from build123d import *

# Parameters (mm, degrees)
SKETCH2_W                  = 23.9522
SKETCH2_H                  = 45.7962
SKETCH2_R                  = 2.2606
SKETCH2_R_2                = 1.016
BOSS_EXTRUDE1_DEPTH        = 6.35
SKETCH4_W                  = 21.4122
SKETCH4_H                  = 43.2562
CUT_EXTRUDE1_DEPTH         = 6.223
CUT_EXTRUDE3_DEPTH         = 2.54
CUT_EXTRUDE5_DEPTH         = 1.27
BOSS_EXTRUDE3_DEPTH        = 6.223
BOSS_EXTRUDE15_OUTLINE_W   = 23.9522
BOSS_EXTRUDE15_OUTLINE_H   = 30.5562
BOSS_EXTRUDE15_OUTLINE_R   = 2.2606
BOSS_EXTRUDE15_OUTLINE_R_2 = 1.016
BOSS_EXTRUDE15_DEPTH       = 1.27
SKETCH14_R                 = 1.190625
CUT_EXTRUDE6_DEPTH         = 1.27


# Read off the part's stored shape, not the designer's step: Boss-Extrude15
with BuildPart() as part:
    # Sketch2 → Boss-Extrude1 (new body)
    with BuildSketch(Plane.XY):
        Rectangle(SKETCH2_W, SKETCH2_H)
        with Locations((0, -8.7249)):
            Circle(SKETCH2_R, mode=Mode.SUBTRACT)
        with Locations((0, 13.4747)):
            Circle(SKETCH2_R_2, mode=Mode.SUBTRACT)
        with BuildLine():
            Line((8.361518313, 5.139100055), (5.725634689, 6.065681687))
            ThreePointArc((5.725634689, 6.065681687), (4.333034634, 5.3975), (5.001216321, 4.004899945))
            Line((5.001216321, 4.004899945), (7.637099945, 3.078318313))
            ThreePointArc((7.637099945, 3.078318313), (9.0297, 3.7465), (8.361518313, 5.139100055))
        make_face(mode=Mode.SUBTRACT)
    extrude(amount=BOSS_EXTRUDE1_DEPTH)

    # Sketch4 → Cut-Extrude1 (cut)
    with BuildSketch(Plane.XY.offset(6.35)):
        Rectangle(SKETCH4_W, SKETCH4_H)
    extrude(amount=-CUT_EXTRUDE1_DEPTH, mode=Mode.SUBTRACT)

    # Sketch6 → Cut-Extrude3 (cut)
    with BuildSketch(Plane.ZY.offset(11.9761)):
        Polygon((4.826, -14.5669), (2.6162, -14.5669), (2.6162, 4.9911), (6.35, 4.9911), (6.35, -18.7833), (4.826, -18.7833), align=None)
    extrude(amount=-CUT_EXTRUDE3_DEPTH, mode=Mode.SUBTRACT)

    # Sketch8 → Cut-Extrude5 (cut)
    with BuildSketch(Plane(origin=(11.9761, 0, 0), x_dir=(0, 0, -1), z_dir=(1, 0, 0))):
        Polygon((-6.35, -18.7833), (-4.826, -18.7833), (-4.826, -14.5669), (-2.8956, -14.5669), (-2.8956, -6.0325), (0, -5.1181), (0, 13.4239), (-6.35, 13.3731), align=None)
    extrude(amount=-CUT_EXTRUDE5_DEPTH, mode=Mode.SUBTRACT)

    # Sketch10 → Boss-Extrude3 (add)
    with BuildSketch(Plane.XY.offset(0.127)):
        with BuildLine():
            ThreePointArc((-10.7061, 20.3581), (-9.808074388, 20.730074388), (-9.4361, 21.6281))
            Line((-9.4361, 21.6281), (-10.7061, 21.6281))
            Line((-10.7061, 21.6281), (-10.7061, 20.3581))
        make_face()
        with BuildLine():
            ThreePointArc((9.4361, 21.6281), (9.808074388, 20.730074388), (10.7061, 20.3581))
            Line((10.7061, 20.3581), (10.7061, 21.6281))
            Line((10.7061, 21.6281), (9.4361, 21.6281))
        make_face()
        with BuildLine():
            ThreePointArc((-9.4361, -21.6281), (-9.808074388, -20.730074388), (-10.7061, -20.3581))
            Line((-10.7061, -20.3581), (-10.7061, -21.6281))
            Line((-10.7061, -21.6281), (-9.4361, -21.6281))
        make_face()
        with BuildLine():
            Line((10.7061, -21.6281), (10.7061, -20.3581))
            ThreePointArc((10.7061, -20.3581), (9.808074388, -20.730074388), (9.4361, -21.6281))
            Line((9.4361, -21.6281), (10.7061, -21.6281))
        make_face()
    extrude(amount=BOSS_EXTRUDE3_DEPTH)

    # Boss-Extrude15 outline → Boss-Extrude15 (add)
    with BuildSketch(Plane(origin=(0, 0, 0), x_dir=(-1, 0, 0), z_dir=(0, 0, -1))):
        with Locations((0, 2.54)):
            Rectangle(BOSS_EXTRUDE15_OUTLINE_W, BOSS_EXTRUDE15_OUTLINE_H)
        with Locations((0, -8.7249)):
            Circle(BOSS_EXTRUDE15_OUTLINE_R, mode=Mode.SUBTRACT)
        with BuildLine():
            ThreePointArc((-7.637099945, 3.078318313), (-9.0297, 3.7465), (-8.361518313, 5.139100055))
            Line((-8.361518313, 5.139100055), (-5.725634689, 6.065681687))
            ThreePointArc((-5.725634689, 6.065681687), (-4.333034634, 5.3975), (-5.001216321, 4.004899945))
            Line((-5.001216321, 4.004899945), (-7.637099945, 3.078318313))
        make_face(mode=Mode.SUBTRACT)
        with Locations((0, 13.4747)):
            Circle(BOSS_EXTRUDE15_OUTLINE_R_2, mode=Mode.SUBTRACT)
    extrude(amount=BOSS_EXTRUDE15_DEPTH)

    # Sketch14 → Cut-Extrude6 (cut)
    with BuildSketch(Plane.ZY.offset(11.9761)):
        with Locations((6.35, 11.528736377)):
            Circle(SKETCH14_R)
    extrude(amount=-CUT_EXTRUDE6_DEPTH, mode=Mode.SUBTRACT)


solid = part.part
CAD build for the part. Positions are in the model's coordinates, mm. A direction names the side the tool comes from. Give positions to 0.01 mm unless a question says otherwise; leave off trailing zeros. Loops run counter-clockwise (first coordinate to the right, second up) from the corner with the lowest first, then second, coordinate; pieces in that order, holes last. Notation, with made-up numbers: M -36.5,63 L 8.5,63 A24 ccw 8.5,85 Z; hole C 39,-13 d4. An arc over 180 degrees is marked long. One line per question, with ' | ' between items. Start each with the question number.
1. Saw through at B-B on y = 15.5. Give the cut face in (x, z), plus the area to 3 significant figures.
2. Two-plate mould, pull along Y, no slides. Class faces 1 (the face through (11, -14.567, 4)), 2 (the face through (0, 17.818, -1)), 3 (the face through (0, -22, 6.35)): pulls with the +Y half, pulls with the -Y half, needs draft (parallel to the pull), parting line crosses it, or undercut.
3. 3-axis set-ups, long thin cutter, end or side, ignore diameter. For faces 4 (the face through (11.976, 0, -1)), 5 (the face through (11.35, -5.582, 1.468)), 6 (the face through (-11, -5, 2.616)), 7 (the face through (-11, -17, 4.826)), 8 (the face through (10.706, 17, 3)): which of +Z, -Z, +X, -X, +Y, -Y reach the whole face in a straight line?
4. Saw through at A-A on x = 0. Give the cut face in (y, z), plus the area to 3 significant figures.
5. Probe L1, parallel to Y at x = 0, z = -0.7; L2, parallel to Y at x = -3.5, z = 0.5; L3, parallel to Y at x = -10.75, z = 5.5. List the from-to ranges inside material, lowest first. Write a range as from..to.
6. Saw through at C-C on z = 3.5. Give the cut face in (x, y), plus the area to 3 significant figures.
7. Flat gauge pins, fed straight in: pin 1 (1.9 mm diameter, centred on y = 3, z = 3.5, fed in from +X); pin 2 (3.5 mm diameter, centred on x = 0, y = 13.47, fed in from +Z); pin 3 (0.6 mm diameter, centred on x = -11, y = -5.5, fed in from +Z). Where does each tip first touch, or does it go through?
8. Saw through at D-D on x = -6. Give the cut face in (y, z), plus the area to 3 significant figures.
Result sheet:
1) outline: M -11.98,-1.27 L 11.98,-1.27 L 11.98,6.35 L 10.71,6.35 L 10.71,0.13 L -10.71,0.13 L -10.71,6.35 L -11.98,6.35 Z | area: 49.3 mm^2
2) face 1: undercut | face 2: pulls with the +Y half | face 3: needs draft
3) face 4: +Z, -Z, +X, +Y, -Y | face 5: +Z, +X | face 6: +Z, -X | face 7: +Z, +X, -X | face 8: +Z
4) outline: M -22.9,0 L -12.74,0 L -12.74,-1.27 L -10.99,-1.27 L -10.99,0.13 L -21.63,0.13 L -21.63,6.35 L -22.9,6.35 Z; M -6.46,-1.27 L 12.46,-1.27 L 12.46,0.13 L -6.46,0.13 Z; M 14.49,-1.27 L 17.82,-1.27 L 17.82,0 L 22.9,0 L 22.9,6.35 L 21.63,6.35 L 21.63,0.13 L 14.49,0.13 Z | area: 51.3 mm^2
5) L1: y = -12.74..-10.99, -6.46..12.46, 14.49..17.82 | L2: y = -22.9..-21.63, 21.63..22.9 | L3: y = -22.9..-18.78, 4.99..10.7, 12.36..22.9
6) outline: M -11.98,-22.9 L 11.98,-22.9 L 11.98,-14.57 L 10.71,-14.57 L 10.71,-20.36 A1.27 ccw 9.44,-21.63 L -9.44,-21.63 A1.27 ccw -10.71,-20.36 L -10.71,-14.57 L -11.98,-14.57 Z; M -11.98,4.99 L -10.71,4.99 L -10.71,20.36 A1.27 ccw -9.44,21.63 L 9.44,21.63 A1.27 ccw 10.71,20.36 L 10.71,13.4 L 11.98,13.4 L 11.98,22.9 L -11.98,22.9 Z | area: 115 mm^2
7) pin 1: stops at x = -10.71 | pin 2: stops at z = 0.13 | pin 3: stops at z = 2.62
8) outline: M -22.9,0 L -12.74,0 L -12.74,-1.27 L 17.82,-1.27 L 17.82,0 L 22.9,0 L 22.9,6.35 L 21.63,6.35 L 21.63,0.13 L -21.63,0.13 L -21.63,6.35 L -22.9,6.35 Z | area: 60.4 mm^2
